from build123d import *

# Parameters (mm, degrees)
SKETCH_1_R          = 1.65
EXTRUDE_1_DEPTH     = 3
SKETCH_2_R          = 1.65
CUT_EXTRUDE_1_DEPTH = 10
SKETCH_3_W          = 41.485680135
SKETCH_3_H          = 40
CUT_EXTRUDE_2_DEPTH = 10


with BuildPart() as part:
    # 草图1 → 凸台-拉伸1 (new body)
    with BuildSketch(Plane(origin=(0, 0, 0), x_dir=(1, 0, 0), z_dir=(0, 1, 0))):
        with BuildLine():
            Line((0, 20), (85, 20))
            ThreePointArc((85, 20), (105, 0), (85, -20))
            Line((85, -20), (0, -20))
            ThreePointArc((0, -20), (-20, 0), (0, 20))
        make_face()
        with Locations(Location((0, 0, 0), (0, 0, 270))):
            Circle(SKETCH_1_R, mode=Mode.SUBTRACT)
        with Locations(Location((85, 0, 0), (0, 0, 270))):
            Circle(SKETCH_1_R, mode=Mode.SUBTRACT)
        with BuildLine():
            Line((26, 15), (26, 7))
            ThreePointArc((26, 7), (24.3, 5.3), (22.6, 7))
            Line((22.6, 7), (22.6, 15))
            ThreePointArc((22.6, 15), (24.3, 16.7), (26, 15))
        make_face(mode=Mode.SUBTRACT)
        with BuildLine():
            Line((26, -7), (26, -15))
            ThreePointArc((26, -15), (24.3, -16.7), (22.6, -15))
            Line((22.6, -15), (22.6, -7))
            ThreePointArc((22.6, -7), (24.3, -5.3), (26, -7))
        make_face(mode=Mode.SUBTRACT)
        with BuildLine():
            Line((59, -7), (59, -15))
            ThreePointArc((59, -15), (60.7, -16.7), (62.4, -15))
            Line((62.4, -15), (62.4, -7))
            ThreePointArc((62.4, -7), (60.7, -5.3), (59, -7))
        make_face(mode=Mode.SUBTRACT)
        with BuildLine():
            Line((59, 15), (59, 7))
            ThreePointArc((59, 7), (60.7, 5.3), (62.4, 7))
            Line((62.4, 7), (62.4, 15))
            ThreePointArc((62.4, 15), (60.7, 16.7), (59, 15))
        make_face(mode=Mode.SUBTRACT)
    extrude(amount=EXTRUDE_1_DEPTH)

    # 草图2 → 切除-拉伸1 (cut)
    with BuildSketch(Plane(origin=(0, 3, 0), x_dir=(1, 0, 0), z_dir=(0, 1, 0))):
        with Locations(Location((24.3, 0, 0), (0, 0, 270))):
            Circle(SKETCH_2_R)
        with Locations(Location((60.7, 0, 0), (0, 0, 270))):
            Circle(SKETCH_2_R)
    extrude(amount=-CUT_EXTRUDE_1_DEPTH, mode=Mode.SUBTRACT)

    # 草图3 → 切除-拉伸2 (cut)
    with BuildSketch(Plane.XZ):
        with Locations((-3.142840067, 0)):
            Rectangle(SKETCH_3_W, SKETCH_3_H)
    extrude(amount=-CUT_EXTRUDE_2_DEPTH, mode=Mode.SUBTRACT)


solid = part.part
CAD build for the part. Positions are in the model's coordinates, mm. A direction names the side the tool comes from. Coordinates: 2 decimals unless noted, no trailing zeros. Loops run counter-clockwise (first coordinate to the right, second up) from the corner with the lowest first, then second, coordinate; pieces in that order, holes last. Notation, with made-up numbers: (7, 37.5) -> (26, 37.5) arc R17 ccw to (26, 56.5) -> close; hole circle Ø8 at (15, 87). An arc over 180 degrees is marked (long way). One line per item, written item: value.
1. Pull direction Z, two halves, no side cores. Call faces 3 (the face through (62, 0, -5)), 4 (the face through (25.69, 1.52, 0.89)), 5 (the face through (105, 1, 0)): pulls with the +Z half, pulls with the -Z half, needs draft (parallel to the pull), parting line crosses it, or undercut.
Answers:
face 3: needs draft
face 4: undercut
face 5: parting line crosses it
2. Flat gauge pins, fed straight in: P1, Ø2, axis at x = 60.7, z = 0, coming from the +Y side; P2, Ø1.5, axis at y = 1.5, z = 10, coming from the +X side; P3, Ø0.9, axis at y = 2, z = -10.5, coming from the +X side. Where does each tip first touch, or does it go through?
Answers:
P1: passes through
P2: stops at x = 102.73
P3: stops at x = 102.29
3. Slice it at D-D on z = 14. Write the cut outline in (x, y), and give its area (3 significant figures).
Answers:
outline: (17.6, 0) -> (22.6, 0) -> (22.6, 3) -> (17.6, 3) -> close; (26, 0) -> (59, 0) -> (59, 3) -> (26, 3) -> close; (62.4, 0) -> (99.28, 0) -> (99.28, 3) -> (62.4, 3) -> close
area: 225 mm^2
4. Which spindle directions (+Z, -Z, +X, -X, +Y, -Y) get a long thin tool onto all of the face, cutting with end or side? Do faces 1 (the face through (60.7, 1.5, -5.3)), 2 (the face through (17.6, 1, 0)). Say none if no direction does.
Answers:
face 1: +Y, -Y
face 2: +Z, -Z, -X, +Y, -Y
5. Drill centre lines: line 1 (X direction, y = 2.4, z = 0); line 2 (X direction, y = 0.95, z = 8.5); line 3 (X direction, y = 2.8, z = -6). Where is each one in solid material? Low to high. Write a range as [from, to].
Answers:
line 1: x = [17.6, 22.65], [25.95, 59.05], [62.35, 83.35], [86.65, 105]
line 2: x = [17.6, 22.6], [26, 59], [62.4, 103.1]
line 3: x = [17.6, 22.93], [25.67, 59.33], [62.07, 104.08]
6. Slice it at A-A on x = 60.7. Write the cut outline in (y, z), and give its area (3 significant figures).
Answers:
outline: (0, -20) -> (3, -20) -> (3, -16.7) -> (0, -16.7) -> close; (0, -5.3) -> (3, -5.3) -> (3, -1.65) -> (0, -1.65) -> close; (0, 1.65) -> (3, 1.65) -> (3, 5.3) -> (0, 5.3) -> close; (0, 16.7) -> (3, 16.7) -> (3, 20) -> (0, 20) -> close
area: 41.7 mm^2
7. Slice it at B-B on z = 0. Write the cut outline in (x, y).
Answers:
outline: (17.6, 0) -> (22.65, 0) -> (22.65, 3) -> (17.6, 3) -> close; (25.95, 0) -> (59.05, 0) -> (59.05, 3) -> (25.95, 3) -> close; (62.35, 0) -> (83.35, 0) -> (83.35, 3) -> (62.35, 3) -> close; (86.65, 0) -> (105, 0) -> (105, 3) -> (86.65, 3) -> close
8. Slice it at C-C on y = 2.1. Write the cut outline in (x, z).
Answers:
outline: (17.6, -20) -> (85, -20) arc R20 ccw to (85, 20) -> (17.6, 20) -> close; hole (22.6, -15) arc R1.7 ccw to (26, -15) -> (26, -7) arc R1.7 ccw to (22.6, -7) -> close; hole (22.6, 7) arc R1.7 ccw to (26, 7) -> (26, 15) arc R1.7 ccw to (22.6, 15) -> close; hole circle Ø3.3 at (24.3, 0); hole (59, -15) arc R1.7 ccw to (62.4, -15) -> (62.4, -7) arc R1.7 ccw to (59, -7) -> close; hole (59, 7) arc R1.7 ccw to (62.4, 7) -> (62.4, 15) arc R1.7 ccw to (59, 15) -> close; hole circle Ø3.3 at (60.7, 0); hole circle Ø3.3 at (85, 0)
